The model under review builds one solid part; all positions refer to its coordinate system, in mm. Face numbers are marked on the shaded views. Coordinates: 2 decimals unless noted, no trailing zeros. Loops run counter-clockwise (first coordinate to the right, second up) from the corner with the lowest first, then second, coordinate; pieces in that order, holes last. Notation, with made-up numbers: (-4.5, 7.25) - (2.5, 7.25) arc R11 cw to (2.5, 24.25) - close; hole circle Ø5 at (86, -11.75). An arc over 180 degrees is marked (long way). Answer in a Markdown table with one row per item. Add a question column.
(1) We need section B-B on z = 38.1. Write out the cut boundary in (x, y) (3 decimals), plus the area to 3 significant figures.
(2) We need section D-D on x = 44.5. Write out the cut boundary in (y, z), plus the area to 3 significant figures.
(3) For line 1 along X through (y, z) = (-7.75, -38.1) (3 decimals); line 2 along X through (y, z) = (-10.25, 42.5) (3 decimals); line 3 along Z through (x, y) = (48, -1.25), list the stretches that pass through material, from the lowest coordinate up.
(4) Mouldability with a two-part tool opening along X and no side actions: class the marked faces 1 and 2 as +X half, -X half, draft (parallel to the pull), parting line (faces both ways), or undercut.
(5) We need section A-A on x = 0. Write out the cut boundary in (y, z), plus the area to 3 significant figures.
(6) We need section C-C on y = -9.5. Give the number of separate pieces and of enclosed holes in the cut face, plus the area to 3 significant figures.
from build123d import *

# Parameters (mm, degrees)
F0_W     = 107.95
F0_H     = 98.425
F0_R     = 6.35
F1_DEPTH = 12.7
F2_D     = 13.49248


with BuildPart() as f1:
    # F0 (on Front) → F1 (new body)
    with BuildSketch(Plane.XZ):
        Rectangle(F0_W, F0_H)
        with Locations((0, 1.5875)):
            Circle(F0_R, mode=Mode.SUBTRACT)
    extrude(amount=F1_DEPTH)

    # F2 (through all)
    with Locations(Plane(origin=(0, 0, 0), x_dir=(1, 0, 0), z_dir=(0, 1, 0))):
        with Locations((-42.8625, -38.1), (42.8625, -38.1), (42.8625, 38.1), (-42.8625, 38.1)):
            Hole(F2_D / 2)


solid = f1.part
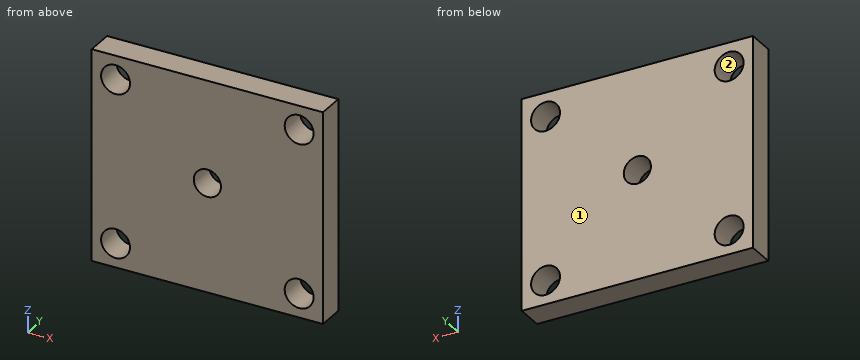
Outcome:
| question | item | result |
|---|---|---|
| 1 | outline | (-53.975, -12.7) - (-49.609, -12.7) - (-49.609, 0) - (-53.975, 0) - close; (-36.116, -12.7) - (36.116, -12.7) - (36.116, 0) - (-36.116, 0) - close; (49.609, -12.7) - (53.975, -12.7) - (53.975, 0) - (49.609, 0) - close |
| 1 | area | 1,030 mm² |
| 2 | outline | (-12.7, -49.21) - (0, -49.21) - (0, -44.64) - (-12.7, -44.64) - close; (-12.7, -31.56) - (0, -31.56) - (0, 31.56) - (-12.7, 31.56) - close; (-12.7, 44.64) - (0, 44.64) - (0, 49.21) - (-12.7, 49.21) - close |
| 2 | area | 918 mm² |
| 3 | line 1 | -53.975 to -49.609, -36.116 to 36.116, 49.609 to 53.975 |
| 3 | line 2 | -53.975 to -47.976, -37.749 to 37.749, 47.976 to 53.975 |
| 3 | line 3 | -49.21 to -42.47, -33.73 to 33.73, 42.47 to 49.21 |
| 4 | face 1 | draft |
| 4 | face 2 | undercut |
| 5 | outline | (-12.7, -49.21) - (0, -49.21) - (0, -4.76) - (-12.7, -4.76) - close; (-12.7, 7.94) - (0, 7.94) - (0, 49.21) - (-12.7, 49.21) - close |
| 5 | area | 1,090 mm² |
| 6 | separate pieces | 1 |
| 6 | enclosed holes | 5 |
| 6 | area | 9,930 mm² |
